Job drawing, mm, ordinate dimensions from the low corner. One solid piece. A direction names the side the tool comes from. Give positions to 0.01 mm unless a question says otherwise; leave off trailing zeros. Order: outer loops, then holes, each group sorted by start corner. A loop starts at its lowest first (then second) coordinate and runs counter-clockwise, first axis right, second up. Notation, with made-up numbers: M 20,-32 L 38,-32 A24 ccw 38,-14 Z; hole C 29,-19 d2. An arc over 180 degrees is marked long. One line per question, with ' | ' between items.
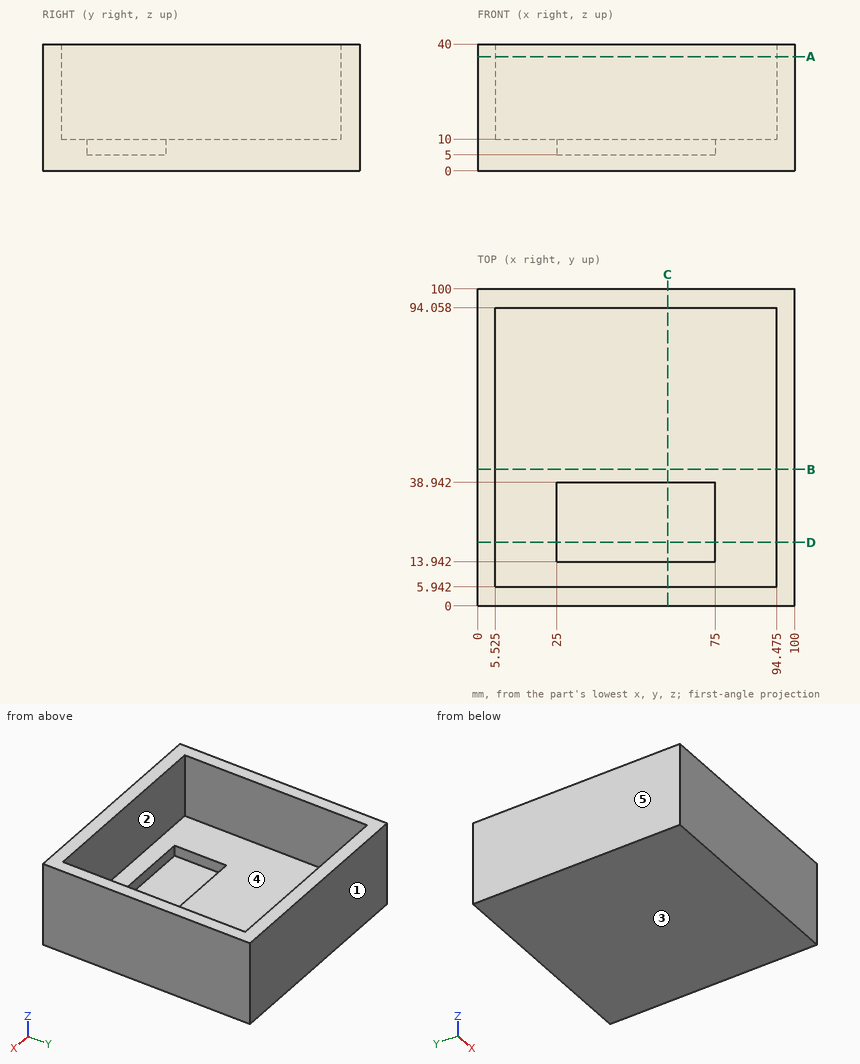
1. Probe L1, parallel to X at y = 88.5, z = 38.5 (1 decimal); L2, parallel to Y at x = 11.5, z = 36; L3, parallel to Z at x = 46.5, y = 23. List the from-to ranges inside material, lowest first. Write a range as from..to.
Worked out:
L1: x = 0..5.5, 94.5..100 | L2: y = 0..5.94, 94.06..100 | L3: z = 0..5
2. Slice it at C-C on x = 60. Give the cut face in (y, z), then the cut area to 3 significant figures.
Worked out:
outline: M 0,0 L 100,0 L 100,40 L 94.06,40 L 94.06,10 L 38.94,10 L 38.94,5 L 13.94,5 L 13.94,10 L 5.94,10 L 5.94,40 L 0,40 Z | area: 1,230 mm2
3. Tool access for the marked faces 1 and 2: list every direction of +Z, -Z, +X, -X, +Y, -Y with a clear straight run to the whole face (end or side of a thin tool).
Worked out:
face 1: +Z, -Z, +X, -X, +Y | face 2: +Z
4. Drop flat-ended pins along their axis: pin 1 (20 mm diameter, centred on x = 60.5, y = 31.5, fed in from +Z); pin 2 (6 mm diameter, centred on x = 87, y = 27.5, fed in from -Z). Give the stop position or say it passes through.
Worked out:
pin 1: stops at z = 10 | pin 2: stops at z = 0
5. Slice it at A-A on z = 36. Give the cut face in (x, y) (1 decimal), then the cut area to 3 significant figures.
Worked out:
outline: M 0,0 L 100,0 L 100,100 L 0,100 Z; hole M 5.5,5.9 L 94.5,5.9 L 94.5,94.1 L 5.5,94.1 Z | area: 2,160 mm2
6. Slice it at D-D on y = 20. Give the cut face in (x, z) (1 decimal).
Worked out:
outline: M 0,0 L 100,0 L 100,40 L 94.5,40 L 94.5,10 L 75,10 L 75,5 L 25,5 L 25,10 L 5.5,10 L 5.5,40 L 0,40 Z
7. Slice it at B-B on y = 43. Give the cut face in (x, z) (1 decimal), then the cut area to 3 significant figures.
Worked out:
outline: M 0,0 L 100,0 L 100,40 L 94.5,40 L 94.5,10 L 5.5,10 L 5.5,40 L 0,40 Z | area: 1,330 mm2
8. Mould opens along X. For the marked faces 3, 4 and 5 say: released by +X, released by -X, zero draft, split by the parting line, or undercut.
Worked out:
face 3: zero draft | face 4: undercut | face 5: released by -X
